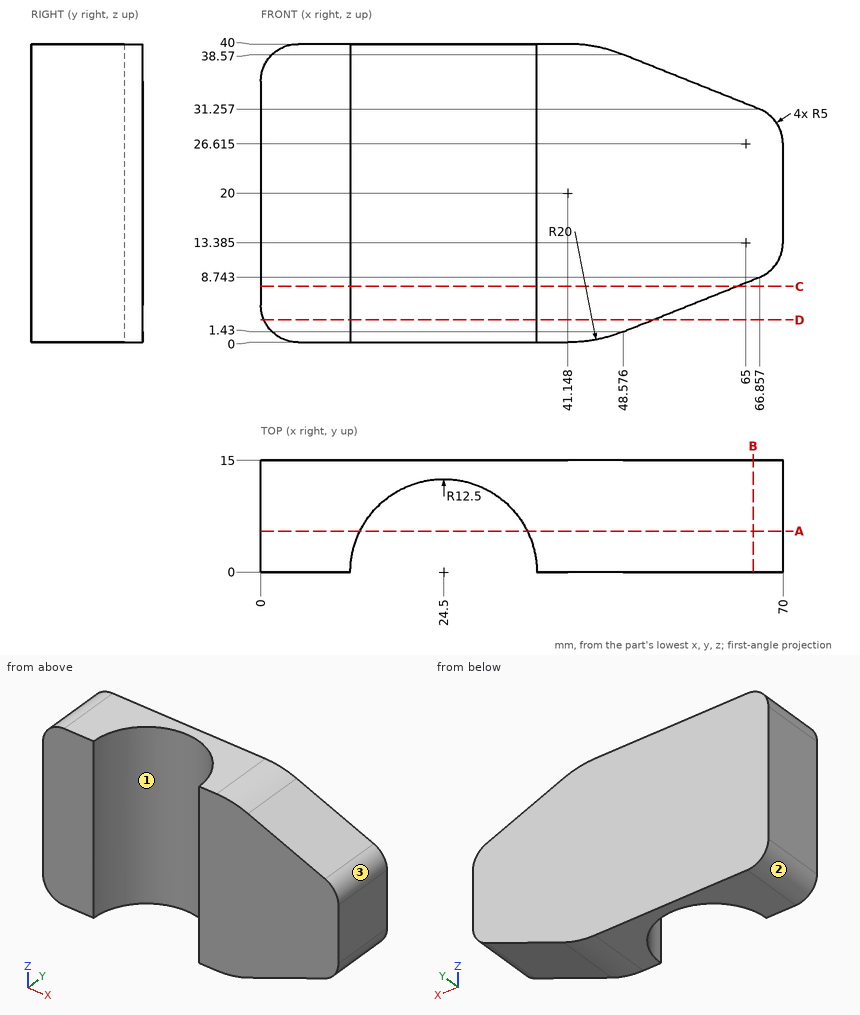
Source: three-view drawing plus pictorial views. Frame: mm from the lowest corner of the part. Round coordinates to 2 decimals unless told otherwise and drop trailing zeros. Loops run counter-clockwise (first coordinate to the right, second up) from the corner with the lowest first, then second, coordinate; pieces in that order, holes last.
1. Mould query, pull axis X, two halves, no side actions, for the marked faces 1, 2 and 3. Classes: released by +X, released by -X, zero draft, split by the parting line, or undercut.
2. Section query A-A on y = 5.5. Output: boundary loops of the cut face in (x, z) (1 decimal), and give its area (3 significant figures).
3. Section query B-B on x = 66. Output: boundary loops of the cut face in (y, z).
4. Ray query, L1, parallel to X at y = 11, z = 20.5 (1 decimal); L2, parallel to X at y = 9.5, z = 14 (1 decimal); L3, parallel to Y at x = 15, z = 21 (1 decimal). Return the intervals inside material, ascending.
5. Section query C-C on z = 7.5. Output: boundary loops of the cut face in (x, y), and give its area (3 significant figures).
6. Contact query for flat-ended pins moving along their axis: pin 1 (1 mm diameter, centred on x = 43, y = 6, fed in from -Z); pin 2 (1.5 mm diameter, centred on y = 2.5, z = 23, fed in from -X); pin 3 (3 mm diameter, centred on x = 51, y = 5.5, fed in from -Z). Output: stop coordinate, or through.
7. Section query D-D on z = 3. Output: boundary loops of the cut face in (x, y).
Answers below:
1. face 1: undercut
1. face 2: released by -X
1. face 3: released by +X
2. outline: (0, 5) arc R5 ccw to (5, 0) - (13.3, 0) - (13.3, 40) - (5, 40) arc R5 ccw to (0, 35) - close; (35.7, 0) - (41.1, 0) arc R20 ccw to (48.6, 1.4) - (66.9, 8.7) arc R5 ccw to (70, 13.4) - (70, 26.6) arc R5 ccw to (66.9, 31.3) - (48.6, 38.6) arc R20 ccw to (41.1, 40) - (35.7, 40) - close
2. area: 1,640 mm2
3. outline: (0, 8.4) - (15, 8.4) - (15, 31.6) - (0, 31.6) - close
4. L1: x = 0 to 18.6, 30.4 to 70
4. L2: x = 0 to 16.4, 32.6 to 70
4. L3: y = 8.1 to 15
5. outline: (0, 0) - (12, 0) arc R12.5 cw to (37, 0) - (63.75, 0) - (63.75, 15) - (0, 15) - close
5. area: 711 mm2
6. pin 1: stops at z = 0.05
6. pin 2: stops at x = 0
6. pin 3: stops at z = 1.8
7. outline: (0.42, 0) - (12, 0) arc R12.5 cw to (37, 0) - (52.5, 0) - (52.5, 15) - (0.42, 15) - close
